Could you check a few things on this model? Use its own coordinates, in mm. A direction names the side the tool comes from. Round coordinates to 2 decimals unless told otherwise and drop trailing zeros. Write each loop counter-clockwise with the first axis right and the second up, starting at its lowest first coordinate (ties: lowest second). Pieces come first, ordered by that corner, then holes. Notation, with made-up numbers: (36.5, 54.5) -> (88.5, 54.5) arc R27 ccw to (88.5, 85.5) -> close; hole circle Ø6 at (-22, 31). An arc over 180 degrees is marked (long way). Answer as CSV lines item,"result". Start each with the question number.
Q1. Imagine slicing it at C-C on y = 29. Please give me the cut outline in (x, z) (3 decimals).
Q2. If I drill on line 1 (Z direction, x = 0, y = 14); line 2 (X direction, y = 6.5, z = 0); line 3 (X direction, y = 15, z = 0) (3 decimals), over which ranges is the centre line in solid material (lowest first)? Write a range as [from, to].
Q3. If we mould it in two halves opening along Z, with no side actions, what happens to faces 1 (the flat face through (67, 31.8, 13)), 2 (the cylindrical face through (-3.905, 18.124, -0.867)), 3 (the flat face through (54, 16, 19.65))? For each: pulls with the +Z half, pulls with the -Z half, needs draft (parallel to the pull), parting line crosses it, or undercut.
Q4. Imagine slicing it at D-D on x = 52. Please give me the cut outline in (y, z) (3 decimals).
Q5. For faces 4 (the flat face through (40, 8, -19.65)), 5 (the flat face through (92, 9, 6.195)), 6 (the flat face through (5, 16.3, 0)), 7 (the flat face through (84.31, 21, -4)), 8 (the flat face through (5, 20, 0)), which set-ups out of +Z, -Z, +X, -X, +Y, -Y let a thin tool reach every point of the face, with its end or its side?
Q6. Imagine slicing it at B-B on z = -22.65. Please give me the cut outline in (x, y).
Q7. Imagine slicing it at A-A on x = 22.65. Please give me the cut outline in (y, z).
Q8. Will these pins go through, and if not, where does the flat tip stop? pin 1 Ø0.6 at (x, z) = (40, -5) entering from +Y; pin 2 Ø3 at (y, z) = (9.5, 12) entering from -X; pin 3 Ø6 at (x, y) = (23.5, 12) entering from +Z.
from build123d import *

# Parameters (mm, degrees)
SKETCH1_R                = 25.65
SKETCH1_R_2              = 19.65
SKETCH1_R_3              = 4
SKETCH1_R_4              = 0.95
SKETCH1_W                = 40.16
SKETCH1_H                = 20.39
BOSS_EXTRUDE2_DEPTH      = 3.7
SKETCH5_R                = 19.65
SKETCH5_W                = 40.16
SKETCH5_H                = 20.39
BOSS_EXTRUDE3_DEPTH      = 28.1
CUT_EXTRUDE1_REACH       = 112.955
SKETCH6_W                = 40.16
SKETCH6_H                = 28.1
CUT_EXTRUDE2_REACH       = 119.305
CUT_EXTRUDE2_END_RADIUS  = 25.65
SKETCH7_W                = 29.863740461
SKETCH7_H                = 10
CUT_EXTRUDE3_DEPTH       = 109.093330622
CUT_EXTRUDE3_DEPTH_BACK  = 109.093330622
SKETCH8_R                = 1.45
SKETCH9_R                = 0.95
CUT_EXTRUDE4_DEPTH       = 12
CUT_EXTRUDE5_DEPTH       = 109.093330622
FILLET1_R                = 2
CUT_EXTRUDE6_DEPTH       = 11.8
BOSS_EXTRUDE4_START      = -3.7
SKETCH14_R               = 19.65
SKETCH14_R_2             = 0.95
SKETCH14_R_3             = 4
BOSS_EXTRUDE4_DEPTH      = 3.7
CUT_EXTRUDE7_START       = -3.7
CUT_EXTRUDE7_OUTLINE_R   = 19.65
CUT_EXTRUDE7_OUTLINE_R_2 = 0.95
CUT_EXTRUDE7_OUTLINE_R_3 = 4
CUT_EXTRUDE7_DEPTH       = 3.7
FILLET2_R                = 2
FILLET3_R                = 2


# Read off the part's stored shape, not the designer's step: Cut-Extrude7
with BuildPart() as part:
    # Sketch1 → Boss-Extrude2 (new body)
    # profile 1 of 6: a face of its own
    with BuildSketch(Plane(origin=(0, 0, 0), x_dir=(1, 0, 0), z_dir=(0, 1, 0))):
        Circle(SKETCH1_R)
        Circle(SKETCH1_R_2, mode=Mode.SUBTRACT)
    # profile 2 of 6: a face of its own
    with BuildSketch(Plane(origin=(0, 0, 0), x_dir=(1, 0, 0), z_dir=(0, 1, 0))):
        Circle(SKETCH1_R_2)
        with Locations(Location((0, 0, 0), (0, 0, 270))):
            Circle(SKETCH1_R_3, mode=Mode.SUBTRACT)
        with Locations(Location((16.6, 0, 0), (0, 0, 270))):
            Circle(SKETCH1_R_4, mode=Mode.SUBTRACT)
        with Locations(Location((0, -16.6, 0), (0, 0, 270))):
            Circle(SKETCH1_R_4, mode=Mode.SUBTRACT)
        with Locations(Location((-16.6, 0, 0), (0, 0, 270))):
            Circle(SKETCH1_R_4, mode=Mode.SUBTRACT)
        with Locations(Location((0, 16.6, 0), (0, 0, 270))):
            Circle(SKETCH1_R_4, mode=Mode.SUBTRACT)
    # profile 3 of 6: a face of its own
    with BuildSketch(Plane(origin=(0, 0, 0), x_dir=(1, 0, 0), z_dir=(0, 1, 0))):
        with BuildLine():
            Line((35.65, 18.695), (91.986875612, 18.695))
            ThreePointArc((91.986875612, 18.695), (83.869462663, 23.847948025), (74.425, 25.65))
            Line((74.425, 25.65), (0, 25.65))
            ThreePointArc((0, 25.65), (18.137288937, 18.137288937), (25.65, 0))
            ThreePointArc((25.65, 0), (18.137288937, -18.137288937), (0, -25.65))
            Line((0, -25.65), (74.425, -25.65))
            ThreePointArc((74.425, -25.65), (83.869462663, -23.847948025), (91.986875612, -18.695))
            Line((91.986875612, -18.695), (35.65, -18.695))
            Line((35.65, -18.695), (35.65, 18.695))
        make_face()
    # profile 4 of 6: a face of its own
    with BuildSketch(Plane(origin=(0, 0, 0), x_dir=(1, 0, 0), z_dir=(0, 1, 0))):
        with BuildLine():
            Line((92.81, -17.886147573), (92.81, 17.886147573))
            ThreePointArc((92.81, 17.886147573), (92.402987293, 18.295203548), (91.986875612, 18.695))
            Line((91.986875612, 18.695), (35.65, 18.695))
            Line((35.65, 18.695), (35.65, -18.695))
            Line((35.65, -18.695), (91.986875612, -18.695))
            ThreePointArc((91.986875612, -18.695), (92.402987293, -18.295203548), (92.81, -17.886147573))
        make_face()
        with Locations((64.23, 0)):
            Rectangle(SKETCH1_W, SKETCH1_H, mode=Mode.SUBTRACT)
    # profile 5 of 6: a face of its own
    with BuildSketch(Plane(origin=(0, 0, 0), x_dir=(1, 0, 0), z_dir=(0, 1, 0))):
        with Locations((64.23, 0)):
            Rectangle(SKETCH1_W, SKETCH1_H)
    # profile 6 of 6: a face of its own
    with BuildSketch(Plane(origin=(0, 0, 0), x_dir=(1, 0, 0), z_dir=(0, 1, 0))):
        with BuildLine():
            ThreePointArc((92.81, -17.886147573), (100.075, 0), (92.81, 17.886147573))
            Line((92.81, 17.886147573), (92.81, -17.886147573))
        make_face()
    extrude(amount=BOSS_EXTRUDE2_DEPTH)

    # Sketch5 → Boss-Extrude3 (add)
    # profile 1 of 4: a face of its own
    with BuildSketch(Plane(origin=(0, 3.7, 0), x_dir=(1, 0, 0), z_dir=(0, 1, 0))):
        with BuildLine():
            ThreePointArc((25.65, 0), (18.137288937, 18.137288937), (0, 25.65))
            ThreePointArc((0, 25.65), (-25.65, 0), (0, -25.65))
            ThreePointArc((0, -25.65), (18.137288937, -18.137288937), (25.65, 0))
        make_face()
        with Locations(Location((0, 0, 0), (0, 0, 270))):
            Circle(SKETCH5_R, mode=Mode.SUBTRACT)
    # profile 2 of 4: a face of its own
    with BuildSketch(Plane(origin=(0, 3.7, 0), x_dir=(1, 0, 0), z_dir=(0, 1, 0))):
        with BuildLine():
            ThreePointArc((92.81, 17.886147573), (92.402987293, 18.295203548), (91.986875612, 18.695))
            Line((91.986875612, 18.695), (35.65, 18.695))
            Line((35.65, 18.695), (35.65, -18.695))
            Line((35.65, -18.695), (91.986875612, -18.695))
            ThreePointArc((91.986875612, -18.695), (92.402987293, -18.295203548), (92.81, -17.886147573))
            Line((92.81, -17.886147573), (92.81, 17.886147573))
        make_face()
        with Locations((64.23, 0)):
            Rectangle(SKETCH5_W, SKETCH5_H, mode=Mode.SUBTRACT)
    # profile 3 of 4: a face of its own
    with BuildSketch(Plane(origin=(0, 3.7, 0), x_dir=(1, 0, 0), z_dir=(0, 1, 0))):
        with BuildLine():
            ThreePointArc((91.986875612, 18.695), (83.869462663, 23.847948025), (74.425, 25.65))
            Line((74.425, 25.65), (0, 25.65))
            ThreePointArc((0, 25.65), (18.137288937, 18.137288937), (25.65, 0))
            ThreePointArc((25.65, 0), (18.137288937, -18.137288937), (0, -25.65))
            Line((0, -25.65), (74.425, -25.65))
            ThreePointArc((74.425, -25.65), (83.869462663, -23.847948025), (91.986875612, -18.695))
            Line((91.986875612, -18.695), (35.65, -18.695))
            Line((35.65, -18.695), (35.65, 18.695))
            Line((35.65, 18.695), (91.986875612, 18.695))
        make_face()
    # profile 4 of 4: a face of its own
    with BuildSketch(Plane(origin=(0, 3.7, 0), x_dir=(1, 0, 0), z_dir=(0, 1, 0))):
        with BuildLine():
            ThreePointArc((92.81, -17.886147573), (100.075, 0), (92.81, 17.886147573))
            Line((92.81, 17.886147573), (92.81, -17.886147573))
        make_face()
    extrude(amount=BOSS_EXTRUDE3_DEPTH)

    # Sketch6 → Cut-Extrude1 (cut, up to next)
    with BuildSketch(Plane.XY.offset(-10.195), mode=Mode.PRIVATE) as cut_extrude1_sk1:
        with Locations((64.23, 17.75)):
            Rectangle(SKETCH6_W, SKETCH6_H)
    cut_extrude1_tool1 = extrude(cut_extrude1_sk1.sketch, amount=-CUT_EXTRUDE1_REACH, mode=Mode.PRIVATE) & part.part
    add(cut_extrude1_tool1.solids().sort_by_distance((64.23, 17.75, -10.195))[0], mode=Mode.SUBTRACT)

    # Cut-Extrude2: up to this cylinder (the profile starts inside it)
    cut_extrude2_end = Plane(origin=(74.425, 8.7, 0), z_dir=(0, -1, 0)) * Cylinder(CUT_EXTRUDE2_END_RADIUS, 290.91, mode=Mode.PRIVATE)
    # Sketch7 → Cut-Extrude2 (cut, up to the surface)
    with BuildSketch(Plane.ZY.offset(-84.31), mode=Mode.PRIVATE) as cut_extrude2_sk1:
        with Locations((-8.736870231, 8.7)):
            Rectangle(SKETCH7_W, SKETCH7_H)
    cut_extrude2_tool1 = extrude(cut_extrude2_sk1.sketch, amount=-CUT_EXTRUDE2_REACH, mode=Mode.PRIVATE) & cut_extrude2_end
    add(cut_extrude2_tool1.solids().sort_by_distance((84.31, 8.7, -8.73687))[0], mode=Mode.SUBTRACT)

    # Sketch8 → Cut-Extrude3 (cut, two sides: drawn at the far end of the back side and taken through both)
    with BuildSketch(Plane(origin=(0, 31.8, 0), x_dir=(1, 0, 0), z_dir=(0, 1, 0)).offset(-CUT_EXTRUDE3_DEPTH_BACK)):
        with Locations(Location((22.65, 0, 0), (0, 0, 270))):
            Circle(SKETCH8_R)
        with Locations(Location((0, -22.65, 0), (0, 0, 270))):
            Circle(SKETCH8_R)
        with Locations(Location((-22.65, 0, 0), (0, 0, 270))):
            Circle(SKETCH8_R)
        with Locations(Location((0, 22.65, 0), (0, 0, 270))):
            Circle(SKETCH8_R)
    extrude(amount=CUT_EXTRUDE3_DEPTH + CUT_EXTRUDE3_DEPTH_BACK, mode=Mode.SUBTRACT)

    # Sketch9 → Cut-Extrude4 (cut)
    with BuildSketch(Plane(origin=(0, 31.8, 0), x_dir=(1, 0, 0), z_dir=(0, 1, 0))):
        with Locations(Location((39.88, -4.95, 0), (0, 0, 270))):
            Circle(SKETCH9_R)
        with Locations(Location((39.88, 4.95, 0), (0, 0, 90))):
            Circle(SKETCH9_R)
        with Locations(Location((87.756875612, -4.95, 0), (0, 0, 90))):
            Circle(SKETCH9_R)
        with Locations(Location((87.756875612, 4.95, 0), (0, 0, 270))):
            Circle(SKETCH9_R)
    extrude(amount=-CUT_EXTRUDE4_DEPTH, mode=Mode.SUBTRACT)

    # Sketch12 → Cut-Extrude5 (cut, through all)
    with BuildSketch(Plane(origin=(0, 31.8, 0), x_dir=(1, 0, 0), z_dir=(0, 1, 0))):
        with BuildLine():
            Line((0, 25.65), (74.425, 25.65))
            ThreePointArc((74.425, 25.65), (83.19711491, 24.103371134), (90.911357997, 19.65))
            Line((90.911357997, 19.65), (16.486357997, 19.65))
            ThreePointArc((16.486357997, 19.65), (8.77211491, 24.103371134), (0, 25.65))
        make_face()
        with BuildLine():
            Line((0, -25.65), (74.425, -25.65))
            ThreePointArc((74.425, -25.65), (83.19711491, -24.103371134), (90.911357997, -19.65))
            Line((90.911357997, -19.65), (16.486357997, -19.65))
            ThreePointArc((16.486357997, -19.65), (8.77211491, -24.103371134), (0, -25.65))
        make_face()
    extrude(amount=-CUT_EXTRUDE5_DEPTH, mode=Mode.SUBTRACT)

    # Fillet1
    fillet1_edges = [part.edges().sort_by_distance(p)[0] for p in [
        (44.15, 17.75, -19.65),
        (84.31, 22.75, -19.65),
    ]]
    fillet(fillet1_edges, radius=FILLET1_R)

    # Sketch13 → Cut-Extrude6 (cut)
    with BuildSketch(Plane(origin=(0, 31.8, 0), x_dir=(1, 0, 0), z_dir=(0, 1, 0))):
        with BuildLine():
            Line((35.65, 19.65), (35.65, -19.65))
            Line((35.65, -19.65), (16.486357997, -19.65))
            ThreePointArc((16.486357997, -19.65), (-25.65, 0), (16.486357997, 19.65))
            Line((16.486357997, 19.65), (35.65, 19.65))
        make_face()
    extrude(amount=-CUT_EXTRUDE6_DEPTH, mode=Mode.SUBTRACT)

    # Sketch14 → Boss-Extrude4 (add)
    with BuildSketch(Plane(origin=(0, 20, 0), x_dir=(1, 0, 0), z_dir=(0, 1, 0)).offset(BOSS_EXTRUDE4_START)):
        with Locations(Location((0, 0, 0), (0, 0, 270))):
            Circle(SKETCH14_R)
        with Locations(Location((16.6, 0, 0), (0, 0, 270))):
            Circle(SKETCH14_R_2, mode=Mode.SUBTRACT)
        with Locations(Location((0, -16.6, 0), (0, 0, 270))):
            Circle(SKETCH14_R_2, mode=Mode.SUBTRACT)
        with Locations(Location((-16.6, 0, 0), (0, 0, 270))):
            Circle(SKETCH14_R_2, mode=Mode.SUBTRACT)
        with Locations(Location((0, 16.6, 0), (0, 0, 270))):
            Circle(SKETCH14_R_2, mode=Mode.SUBTRACT)
        with Locations(Location((0, 0, 0), (0, 0, 270))):
            Circle(SKETCH14_R_3, mode=Mode.SUBTRACT)
    extrude(amount=BOSS_EXTRUDE4_DEPTH)

    # Cut-Extrude7 outline → Cut-Extrude7 (cut)
    with BuildSketch(Plane.XZ.offset(CUT_EXTRUDE7_START)):
        Circle(CUT_EXTRUDE7_OUTLINE_R)
        with Locations((0, -16.6)):
            Circle(CUT_EXTRUDE7_OUTLINE_R_2, mode=Mode.SUBTRACT)
        with Locations((-16.6, 0)):
            Circle(CUT_EXTRUDE7_OUTLINE_R_2, mode=Mode.SUBTRACT)
        Circle(CUT_EXTRUDE7_OUTLINE_R_3, mode=Mode.SUBTRACT)
        with Locations((16.6, 0)):
            Circle(CUT_EXTRUDE7_OUTLINE_R_2, mode=Mode.SUBTRACT)
        with Locations((0, 16.6)):
            Circle(CUT_EXTRUDE7_OUTLINE_R_2, mode=Mode.SUBTRACT)
    extrude(amount=CUT_EXTRUDE7_DEPTH, mode=Mode.SUBTRACT)

    # Fillet2
    fillet2_edges = [part.edges().sort_by_distance(p)[0] for p in [
        (35.65, 25.9, -19.65),
        (35.65, 25.9, 19.65),
    ]]
    fillet(fillet2_edges, radius=FILLET2_R)

    # Fillet3
    fillet3_edges = [part.edges().sort_by_distance(p)[0] for p in [
        (35.65, 20, 0),
        (36.235786438, 20, -19.064213562),
        (36.235786438, 20, 19.064213562),
    ]]
    fillet(fillet3_edges, radius=FILLET3_R)


solid = part.part
Checks:
1,outline,"(35.65, -17.65) arc R2 ccw to (37.65, -19.65) -> (42.15, -19.65) arc R2 ccw to (44.15, -17.65) -> (44.15, 10.195) -> (84.31, 10.195) -> (84.31, -17.65) arc R2 ccw to (86.31, -19.65) -> (90.911, -19.65) arc R25.65 ccw to (91.987, -18.695) arc R25.65 ccw to (92.81, -17.886) arc R25.65 ccw to (92.81, 17.886) arc R25.65 ccw to (91.987, 18.695) arc R25.65 ccw to (90.911, 19.65) -> (37.65, 19.65) arc R2 ccw to (35.65, 17.65) -> close; hole circle Ø1.9 at (39.88, -4.95); hole circle Ø1.9 at (39.88, 4.95); hole circle Ø1.9 at (87.757, -4.95); hole circle Ø1.9 at (87.757, 4.95)"
2,line 1,"[-25.65, -24.1], [-21.2, -19.65], [19.65, 21.2], [24.1, 25.65]"
2,line 2,"[-25.65, -24.1], [-21.2, -19.65], [19.65, 21.2], [24.1, 44.15]"
2,line 3,"[-25.65, -24.1], [-21.2, -19.65], [19.65, 21.2], [24.1, 44.15], [84.31, 100.075]"
3,face 1,"needs draft"
3,face 2,"undercut"
3,face 3,"pulls with the +Z half"
4,outline,"(0, -19.65) -> (3.7, -19.65) -> (3.7, 10.195) -> (31.8, 10.195) -> (31.8, 19.65) -> (0, 19.65) -> close"
5,face 4,"-Z, +X, +Y, -Y"
5,face 5,"-Z, +X"
5,face 6,"-Y"
5,face 7,"-Z, +Y"
5,face 8,"+Z, -Z, -X, +Y"
6,outline,"(-12.04, 0) -> (-1.45, 0) -> (-1.45, 20) -> (-12.04, 20) -> close; (1.45, 0) -> (12.04, 0) -> (12.04, 20) -> (1.45, 20) -> close"
7,outline,"(0, -19.65) -> (20, -19.65) -> (20, -1.45) -> (0, -1.45) -> close; (0, 1.45) -> (20, 1.45) -> (20, 19.65) -> (0, 19.65) -> close"
8,pin 1,"y = 19.8"
8,pin 2,"x = -23.4"
8,pin 3,"z = 19.65"
